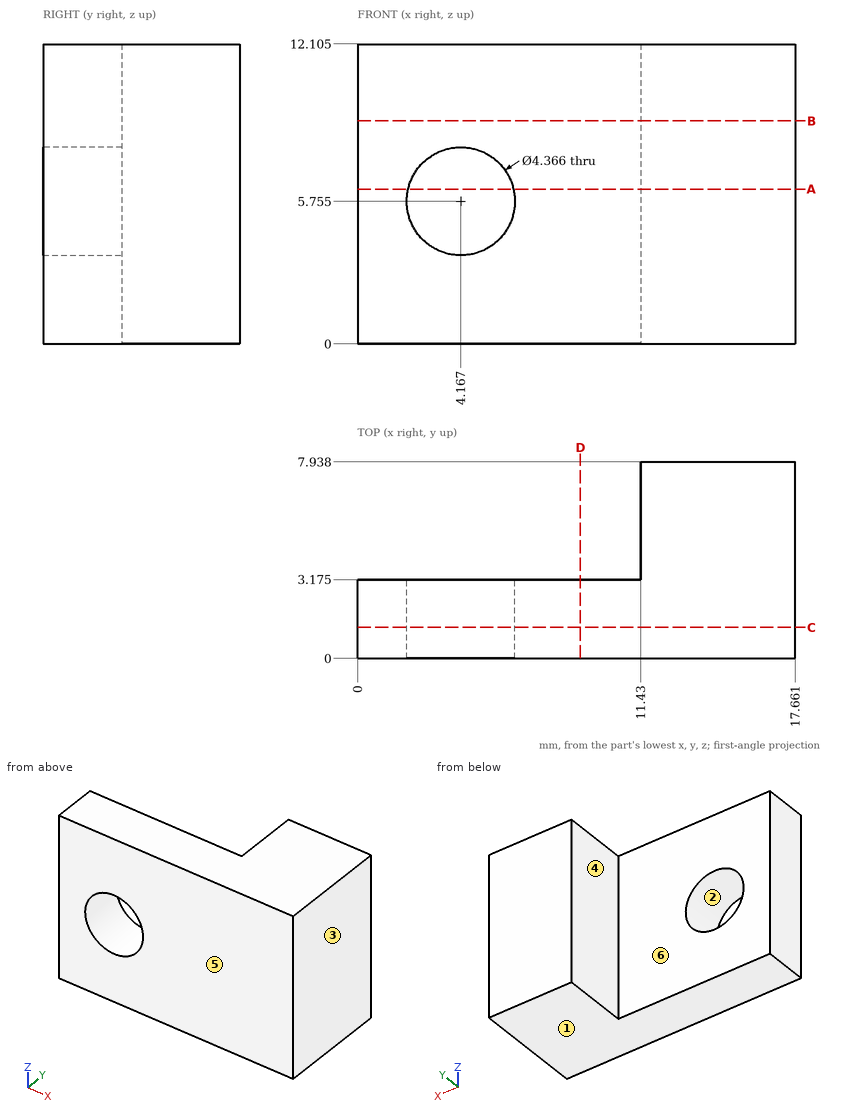
The drawing under review shows one solid part. Ordinate dimensions are in mm from its lowest x, y, z. A direction names the side the tool comes from. Round coordinates to 2 decimals unless told otherwise and drop trailing zeros. Loops run counter-clockwise (first coordinate to the right, second up) from the corner with the lowest first, then second, coordinate; pieces in that order, holes last. Notation, with made-up numbers: (65, -11) -> (109, -11) arc R23 cw to (109, 0) -> close; hole circle Ø6 at (61, 57). An arc over 180 degrees is marked (long way). One line per question, with ' | ' between items. Start each with the question number.
Item 1: Add section A-A, the plane z = 6.25. Write out the cut boundary in (x, y) (1 decimal).
Item 2: Add section B-B, the plane z = 9. Write out the cut boundary in (x, y) (1 decimal).
Item 3: Wall thickness on line 1 along Y through (x, z) = (2.5, 1.5) (1 decimal); line 2 along X through (y, z) = (7.5, 10.5); line 3 along X through (y, z) = (0.5, 7.25) (1 decimal): over which ranges is each line inside the solid? List them lowest first. Write a range as [from, to].
Item 4: Draft analysis for pull direction X (two halves, no side actions). For the marked faces 1, 2, 3 and 4, state which applies: +X half, -X half, draft (parallel to the pull), parting line (faces both ways), or undercut.
Item 5: Add section D-D, the plane x = 9. Write out the cut boundary in (y, z) (1 decimal).
Item 6: Machinability: for the marked faces 5 and 6, which of the approach directions +Z, -Z, +X, -X, +Y, -Y give a long, thin tool a straight path to every point of the face, cutting with its end or side? Answer none if there is none.
Item 7: Add section C-C, the plane y = 1.25. Write out the cut boundary in (x, z) (1 decimal).
Item 8: For pin 1 (2 mm diameter, centred on y = 4.5, z = 4.5, fed in from -X); pin 2 (4 mm diameter, centred on x = 4.17, z = 5.75, fed in from -Y), all flat-tipped, find the tip position at first contact; note any pin that passes through.
Return value:
1) outline: (0, 0) -> (2, 0) -> (2, 3.2) -> (0, 3.2) -> close; (6.3, 0) -> (17.7, 0) -> (17.7, 7.9) -> (11.4, 7.9) -> (11.4, 3.2) -> (6.3, 3.2) -> close
2) outline: (0, 0) -> (17.7, 0) -> (17.7, 7.9) -> (11.4, 7.9) -> (11.4, 3.2) -> (0, 3.2) -> close
3) line 1: y = [0, 3.2] | line 2: x = [11.43, 17.66] | line 3: x = [0, 2.6], [5.8, 17.7]
4) face 1: draft | face 2: undercut | face 3: +X half | face 4: -X half
5) outline: (0, 0) -> (3.2, 0) -> (3.2, 12.1) -> (0, 12.1) -> close
6) face 5: +Z, -Z, +X, -X, -Y | face 6: +Z, -Z, -X, +Y
7) outline: (0, 0) -> (17.7, 0) -> (17.7, 12.1) -> (0, 12.1) -> close; hole circle Ø4.4 at (4.2, 5.8)
8) pin 1: stops at x = 11.43 | pin 2: passes through
